```python
from build123d import *

# Parameters (mm, degrees)
F0_W     = 635
F0_H     = 457.2
F1_DEPTH = 914.4
F2_T     = -2.54
F3_W     = 629.92
F3_H     = 3.175
F4_DEPTH = 1219.2
F5_R     = 50.8


with BuildPart() as f1:
    # F0 (on Top) → F1 (new body)
    with BuildSketch(Plane.XY):
        Rectangle(F0_W, F0_H)
    extrude(amount=F1_DEPTH)

    # F2
    f2_openings = [f1.faces().sort_by_distance(p)[0] for p in [
        (0, 0, 914.4),
    ]]
    offset(amount=F2_T, openings=f2_openings)

    # F3 (on face) → F4 (join)
    with BuildSketch(Plane.XY.offset(2.54)):
        Rectangle(F3_W, F3_H)
    extrude(amount=F4_DEPTH)

    # F5
    f5_edges = [f1.edges().sort_by_distance(p)[0] for p in [
        (314.96, 0, 1221.74),
        (-314.96, 0, 1221.74),
    ]]
    fillet(f5_edges, radius=F5_R)


solid = f1.part
```
The model under review builds one solid part; all positions refer to its coordinate system, in mm. A direction names the side the tool comes from. Give positions to 0.01 mm unless a question says otherwise; leave off trailing zeros. Write each loop counter-clockwise with the first axis right and the second up, starting at its lowest first coordinate (ties: lowest second). Pieces come first, ordered by that corner, then holes.
(1) Consider section D-D, the plane z = 967. Give the boundary of the cut face in (x, y), and give its area (3 significant figures).
(2) Tool access review of faces 4 (the flat face through (317.5, -3, 451)), 5 (the flat face through (-4, -1.588, 604)): name each direction out of +Z, -Z, +X, -X, +Y, -Y from which nothing blocks a thin tool from reaching the whole face with its end or side.
(3) The part is to be moulded in two halves that separate along Y. For faces 1 (the cylindrical face through (-300.474, 0.022, 1206.464)), 2 (the flat face through (-314.96, -115, 452)), 3 (the flat face through (-4, -228.6, 451)), say which applies: released by +Y, released by -Y, zero draft, split by the parting line, or undercut.
(4) Consider section C-C, the plane y = -135. Give the boundary of the cut face in (x, z).
(5) For P1, Ø5, axis at x = 69.5, y = 18, coming from the +Z side; P2, Ø3.5, axis at y = -0.5, z = 1083.5, coming from the +X side; P3, Ø1, axis at y = 0, z = 1101.5, coming from the -X side, all flat-tipped, find the tip position at first contact; note any pin that passes through.
(6) Consider section B-B, the plane x = 208.5. Give the boundary of the cut face in (y, z).
(7) Consider section A-A, the plane z = 410. Give the boundary of the cut face in (x, y).
(8) To check wall thickness, follow L1, parallel to Y at x = 4, z = 519; L2, parallel to X at y = -121, z = 142.5; L3, parallel to Z at x = -145, y = 106. State the ranges of each line that lie inside material, in increasing order.
Returned:
1. outline: (-314.96, -1.59) - (314.96, -1.59) - (314.96, 1.59) - (-314.96, 1.59) - close
1. area: 2,000 mm2
2. face 4: +Z, -Z, +X, +Y, -Y
2. face 5: +Z
3. face 1: zero draft
3. face 2: undercut
3. face 3: released by -Y
4. outline: (-317.5, 0) - (317.5, 0) - (317.5, 914.4) - (314.96, 914.4) - (314.96, 2.54) - (-314.96, 2.54) - (-314.96, 914.4) - (-317.5, 914.4) - close
5. P1: stops at z = 2.54
5. P2: stops at x = 314.96
5. P3: stops at x = -314.96
6. outline: (-228.6, 0) - (228.6, 0) - (228.6, 914.4) - (226.06, 914.4) - (226.06, 2.54) - (1.59, 2.54) - (1.59, 1221.74) - (-1.59, 1221.74) - (-1.59, 2.54) - (-226.06, 2.54) - (-226.06, 914.4) - (-228.6, 914.4) - close
7. outline: (-317.5, -228.6) - (317.5, -228.6) - (317.5, 228.6) - (-317.5, 228.6) - close; hole (-314.96, -226.06) - (314.96, -226.06) - (314.96, -1.59) - (-314.96, -1.59) - close; hole (-314.96, 1.59) - (314.96, 1.59) - (314.96, 226.06) - (-314.96, 226.06) - close
8. L1: y = -228.6 to -226.06, -1.59 to 1.59, 226.06 to 228.6
8. L2: x = -317.5 to -314.96, 314.96 to 317.5
8. L3: z = 0 to 2.54
